Geometry check sheet. Reference: drawing and pictorial views, mm from the part's lowest x, y, z. A direction names the side the tool comes from. Round coordinates to 2 decimals unless told otherwise and drop trailing zeros. Write each loop counter-clockwise with the first axis right and the second up, starting at its lowest first coordinate (ties: lowest second). Pieces come first, ordered by that corner, then holes. Notation, with made-up numbers: M 27.5,-10 L 85.5,-10 A4 cw 85.5,-5 Z; hole C 71.5,-39 d11. An arc over 180 degrees is marked long. Put each result on its own line as item: value. Start each with the question number.
(1) Tool access check on the marked faces 4, 5 and 6. Record the directions out of +Z, -Z, +X, -X, +Y, -Y that give a thin tool (end or side, any length) a straight path to the whole face; none if there is none.
(2) Section check C-C on z = 4.2. Record the cut outline in (x, y).
(3) Mould release check, pull along X, two halves, no side actions. Record for the marked faces 1, 2 and 3: pulls with the +X half, pulls with the -X half, needs draft (parallel to the pull), parting line crosses it, or undercut.
(4) Gauge pin test, flat end, axial feed: pin 1 (1 mm diameter, centred on y = 4.5, z = 0.5, fed in from -X). Record the tip position at first contact, or that the pin passes through.
(5) Material ranges on probe 1 along Y at (x, z) = (6.5, 0.3); probe 2 along Z at (x, y) = (3.5, 2.25); probe 3 along Y at (x, z) = (6.5, 1.7), recorded low to high.
(6) Section check A-A on x = 6.5. Record the cut outline in (y, z).
(7) Section check D-D on y = 10.5. Record the cut outline in (x, z), then the cut area to 3 significant figures.
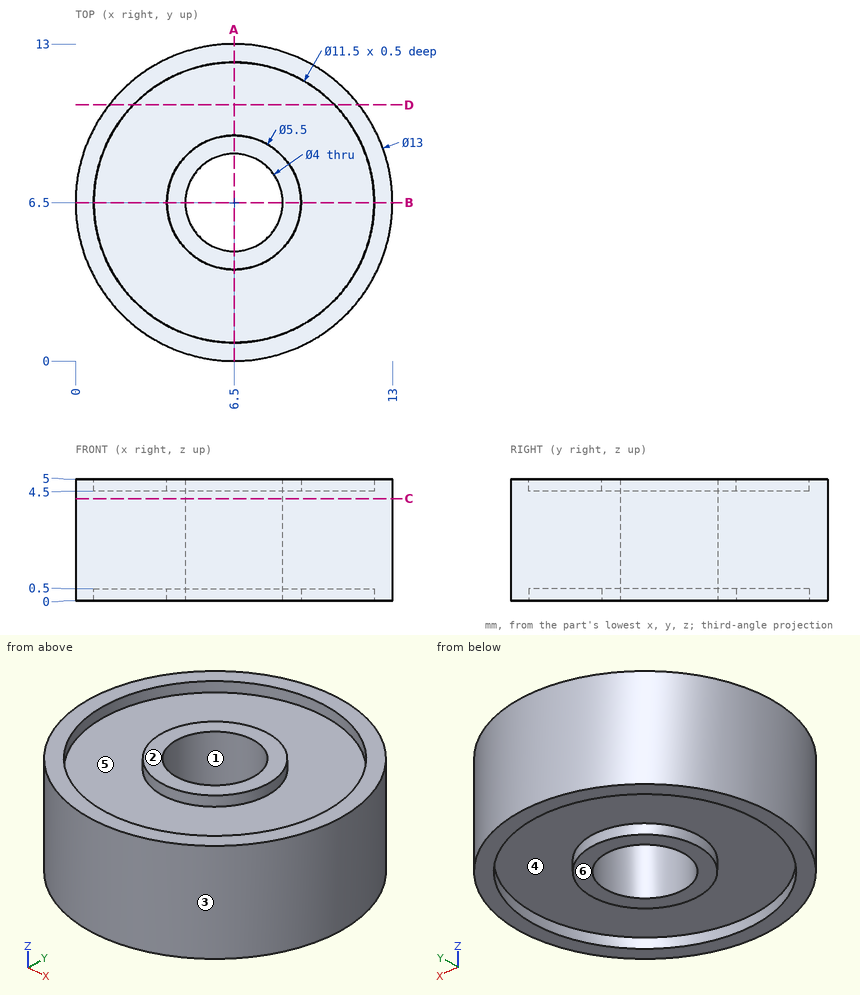
Answers follow:
1. face 4: -Z
1. face 5: +Z
1. face 6: -Z, +X, -X, +Y, -Y
2. outline: C 6.5,6.5 d13; hole C 6.5,6.5 d4
3. face 1: undercut
3. face 2: needs draft
3. face 3: parting line crosses it
4. pin 1: stops at x = 0.18
5. probe 1: y = 0 to 0.75, 3.75 to 4.5, 8.5 to 9.25, 12.25 to 13
5. probe 2: z = 0.5 to 4.5
5. probe 3: y = 0 to 4.5, 8.5 to 13
6. outline: M 0,0 L 0.75,0 L 0.75,0.5 L 3.75,0.5 L 3.75,0 L 4.5,0 L 4.5,5 L 3.75,5 L 3.75,4.5 L 0.75,4.5 L 0.75,5 L 0,5 Z; M 8.5,0 L 9.25,0 L 9.25,0.5 L 12.25,0.5 L 12.25,0 L 13,0 L 13,5 L 12.25,5 L 12.25,4.5 L 9.25,4.5 L 9.25,5 L 8.5,5 Z
7. outline: M 1.38,0 L 2.37,0 L 2.37,0.5 L 10.63,0.5 L 10.63,0 L 11.62,0 L 11.62,5 L 10.63,5 L 10.63,4.5 L 2.37,4.5 L 2.37,5 L 1.38,5 Z
7. area: 43.0 mm^2
